Check sheet for the modelled part. Datum: model origin and axes. Units: mm. A direction names the side the tool comes from. Give positions to 0.01 mm unless a question says otherwise; leave off trailing zeros. Order: outer loops, then holes, each group sorted by start corner. A loop starts at its lowest first (then second) coordinate and runs counter-clockwise, first axis right, second up.
from build123d import *

# Parameters (mm, degrees)
SKETCH1_W            = 40
SKETCH1_H            = 20
BOSS_EXTRUDE1_DEPTH  = 35.9
SKETCH2_W            = 20
SKETCH2_H            = 2
BOSS_EXTRUDE2_DEPTH  = 7
SKETCH3_W            = 7
SKETCH3_H            = 1
BOSS_EXTRUDE3_DEPTH  = 1
CUT_EXTRUDE1_REACH   = 55.852
SKETCH4_R            = 2
FILLET1_R            = 1
CUT_EXTRUDE2_DEPTH   = 11
FILLET1_OF_MIRROR1_R = 1
SKETCH6_W            = 39
SKETCH6_H            = 19
BOSS_EXTRUDE4_DEPTH  = 0.5
BOSS_EXTRUDE5_DEPTH  = 2
SKETCH8_R            = 10
BOSS_EXTRUDE6_DEPTH  = 2.5
SKETCH9_R            = 6
BOSS_EXTRUDE7_DEPTH  = 1
SKETCH10_R           = 5
BOSS_EXTRUDE8_DEPTH  = 0.5
SKETCH11_W           = 10
SKETCH11_H           = 17
BOSS_EXTRUDE9_DEPTH  = 0.5
SKETCH12_R           = 3
BOSS_EXTRUDE10_DEPTH = 4
SKETCH13_W           = 6
SKETCH13_H           = 4
BOSS_EXTRUDE11_DEPTH = 1
SKETCH14_W           = 5.6
SKETCH14_H           = 3.6
SKETCH14_W_2         = 5
SKETCH14_H_2         = 3
BOSS_EXTRUDE12_DEPTH = 4


with BuildPart() as part:
    # Sketch1 → Boss-Extrude1 (new body)
    with BuildSketch(Plane(origin=(0, 0, 0), x_dir=(1, 0, 0), z_dir=(0, 1, 0))):
        with Locations((20, 10)):
            Rectangle(SKETCH1_W, SKETCH1_H)
    extrude(amount=BOSS_EXTRUDE1_DEPTH)

    # Sketch2 → Boss-Extrude2 (add)
    with BuildSketch(Plane(origin=(0, 0, 0), x_dir=(0, 0, -1), z_dir=(1, 0, 0))):
        with Locations((10, 29)):
            Rectangle(SKETCH2_W, SKETCH2_H)
    boss_extrude2 = extrude(amount=-BOSS_EXTRUDE2_DEPTH)

    # Sketch3 → Boss-Extrude3 (add)
    with BuildSketch(Plane(origin=(0, 30, 0), x_dir=(1, 0, 0), z_dir=(0, 1, 0))):
        with Locations((-3.5, 10)):
            Rectangle(SKETCH3_W, SKETCH3_H)
    boss_extrude3 = extrude(amount=BOSS_EXTRUDE3_DEPTH)

    # Sketch4 → Cut-Extrude1 (cut, up to next)
    with BuildSketch(Plane(origin=(0, 30, 0), x_dir=(1, 0, 0), z_dir=(0, 1, 0)), mode=Mode.PRIVATE) as cut_extrude1_sk1:
        with Locations((-5.2, 15.25)):
            Circle(SKETCH4_R)
    cut_extrude1_tool1 = extrude(cut_extrude1_sk1.sketch, amount=-CUT_EXTRUDE1_REACH, mode=Mode.PRIVATE) & part.part
    # Sketch4 → Cut-Extrude1 (cut, up to next)
    with BuildSketch(Plane(origin=(0, 30, 0), x_dir=(1, 0, 0), z_dir=(0, 1, 0)), mode=Mode.PRIVATE) as cut_extrude1_sk2:
        with Locations((-5.2, 4.75)):
            Circle(SKETCH4_R)
    cut_extrude1_tool2 = extrude(cut_extrude1_sk2.sketch, amount=-CUT_EXTRUDE1_REACH, mode=Mode.PRIVATE) & part.part
    cut_extrude1_1 = cut_extrude1_tool1.solids().sort_by_distance((-5.2, 30, -15.25))[0]
    add(cut_extrude1_1, mode=Mode.SUBTRACT)
    cut_extrude1_2 = cut_extrude1_tool2.solids().sort_by_distance((-5.2, 30, -4.75))[0]
    add(cut_extrude1_2, mode=Mode.SUBTRACT)
    cut_extrude1 = cut_extrude1_1 + cut_extrude1_2  # Cut-Extrude1 as one shape, for the pattern or mirror that repeats it

    # Fillet1
    fillet1_edges = [part.edges().sort_by_distance(p)[0] for p in [
        (-7, 29, 0),
        (-7, 29, -20),
    ]]
    fillet(fillet1_edges, radius=FILLET1_R)

    # Sketch5 → Cut-Extrude2 (cut)
    with BuildSketch(Plane.XY.offset(-9.5)):
        Polygon((-7, 30), (0, 31), (-7, 31), align=None)
    cut_extrude2 = extrude(amount=-CUT_EXTRUDE2_DEPTH, mode=Mode.SUBTRACT)

    # Mirror1: Boss-Extrude2, Boss-Extrude3, Cut-Extrude1, Cut-Extrude2 across plane
    add(boss_extrude2.mirror(Plane(origin=(20, 0, 0), x_dir=(0, 0, 1), z_dir=(1, 0, 0))))
    add(boss_extrude3.mirror(Plane(origin=(20, 0, 0), x_dir=(0, 0, 1), z_dir=(1, 0, 0))))
    add(cut_extrude1.mirror(Plane(origin=(20, 0, 0), x_dir=(0, 0, 1), z_dir=(1, 0, 0))), mode=Mode.SUBTRACT)
    add(cut_extrude2.mirror(Plane(origin=(20, 0, 0), x_dir=(0, 0, 1), z_dir=(1, 0, 0))), mode=Mode.SUBTRACT)

    # Fillet1 of Mirror1
    fillet1_of_mirror1_edges = [part.edges().sort_by_distance(p)[0] for p in [
        (47, 29, 0),
        (47, 29, -20),
    ]]
    fillet(fillet1_of_mirror1_edges, radius=FILLET1_OF_MIRROR1_R)

    # Sketch6 → Boss-Extrude4 (add)
    with BuildSketch(Plane(origin=(0, 35.9, 0), x_dir=(1, 0, 0), z_dir=(0, 1, 0))):
        with Locations((20, 10)):
            Rectangle(SKETCH6_W, SKETCH6_H)
    extrude(amount=BOSS_EXTRUDE4_DEPTH)

    # Sketch7 → Boss-Extrude5 (add)
    with BuildSketch(Plane(origin=(0, 36.4, 0), x_dir=(1, 0, 0), z_dir=(0, 1, 0))):
        with BuildLine():
            Line((5.5, 19.5), (30.5, 19.5))
            Line((30.5, 19.5), (30.5, 0.5))
            Line((30.5, 0.5), (5.5, 0.5))
            Line((5.5, 0.5), (5.5, 6.717431229))
            ThreePointArc((5.5, 6.717431229), (4.518757843, 10), (5.5, 13.282568771))
            Line((5.5, 13.282568771), (5.5, 19.5))
        make_face()
    extrude(amount=BOSS_EXTRUDE5_DEPTH)

    # Sketch8 → Boss-Extrude6 (add)
    with BuildSketch(Plane(origin=(0, 38.4, 0), x_dir=(1, 0, 0), z_dir=(0, 1, 0))):
        with Locations((30, 10)):
            Circle(SKETCH8_R)
    extrude(amount=-BOSS_EXTRUDE6_DEPTH)

    # Sketch9 → Boss-Extrude7 (add)
    with BuildSketch(Plane(origin=(0, 38.4, 0), x_dir=(1, 0, 0), z_dir=(0, 1, 0))):
        with Locations(Location((30, 10, 0), (0, 0, 270))):
            Circle(SKETCH9_R)
    extrude(amount=BOSS_EXTRUDE7_DEPTH)

    # Sketch10 → Boss-Extrude8 (add)
    with BuildSketch(Plane(origin=(0, 39.4, 0), x_dir=(1, 0, 0), z_dir=(0, 1, 0))):
        with Locations(Location((30, 10, 0), (0, 0, 270))):
            Circle(SKETCH10_R)
    extrude(amount=BOSS_EXTRUDE8_DEPTH)

    # Sketch11 → Boss-Extrude9 (add)
    with BuildSketch(Plane(origin=(0, 38.4, 0), x_dir=(1, 0, 0), z_dir=(0, 1, 0))):
        with BuildLine():
            Line((5.5, 0.5), (17.5, 0.5))
            Line((17.5, 0.5), (17.5, 8.5))
            ThreePointArc((17.5, 8.5), (19, 10), (17.5, 11.5))
            Line((17.5, 11.5), (17.5, 19.5))
            Line((17.5, 19.5), (5.5, 19.5))
            Line((5.5, 19.5), (5.5, 0.5))
        make_face()
        with Locations((11.5, 10)):
            Rectangle(SKETCH11_W, SKETCH11_H, mode=Mode.SUBTRACT)
    extrude(amount=BOSS_EXTRUDE9_DEPTH)

    # Sketch12 → Boss-Extrude10 (add)
    with BuildSketch(Plane(origin=(0, 39.9, 0), x_dir=(1, 0, 0), z_dir=(0, 1, 0))):
        with Locations(Location((30, 10, 0), (0, 0, 270))):
            Circle(SKETCH12_R)
    extrude(amount=BOSS_EXTRUDE10_DEPTH)

    # Sketch13 → Boss-Extrude11 (add)
    with BuildSketch(Plane(origin=(40, 0, 0), x_dir=(0, 0, -1), z_dir=(1, 0, 0))):
        with Locations((10, 5)):
            Rectangle(SKETCH13_W, SKETCH13_H)
    extrude(amount=BOSS_EXTRUDE11_DEPTH)

    # Sketch14 → Boss-Extrude12 (add)
    with BuildSketch(Plane(origin=(41, 0, 0), x_dir=(0, 0, -1), z_dir=(1, 0, 0))):
        with Locations((10, 5)):
            Rectangle(SKETCH14_W, SKETCH14_H)
        with Locations((10, 5)):
            Rectangle(SKETCH14_W_2, SKETCH14_H_2, mode=Mode.SUBTRACT)
    extrude(amount=BOSS_EXTRUDE12_DEPTH)


solid = part.part
1) Section check C-C, the plane x = 32. Record the cut outline in (y, z).
Recorded:
outline: (0, -20) - (35.9, -20) - (35.9, -19.8) - (38.4, -19.8) - (38.4, -15.66) - (39.4, -15.66) - (39.4, -14.58) - (39.9, -14.58) - (39.9, -12.24) - (43.9, -12.24) - (43.9, -7.76) - (39.9, -7.76) - (39.9, -5.42) - (39.4, -5.42) - (39.4, -4.34) - (38.4, -4.34) - (38.4, -0.2) - (35.9, -0.2) - (35.9, 0) - (0, 0) - close
2) Draft check along X on faces 1 (the face through (24.677, 38.893, -7.231)), 2 (the face through (37.9, 35.9, -0.2)), 3 (the face through (0, 33, -10)), 4 (the face through (19, 38.6, -10)). Enter one of: +X half, -X half, draft (parallel to the pull), parting line (faces both ways), or undercut.
Recorded:
face 1: undercut
face 2: draft
face 3: -X half
face 4: undercut
3) Set-up check for faces 5 (the face through (43, 5, -7.5)), 6 (the face through (43, 30, -5)), 7 (the face through (43, 5, -12.8)): record each of +Z, -Z, +X, -X, +Y, -Y from which the full face is reachable in a straight line by a thin tool's end or side.
Recorded:
face 5: +X
face 6: +Z, +X, +Y
face 7: -Z, +X, -Y
4) Section check A-A, the plane x = 38. Record the cut outline in (y, z).
Recorded:
outline: (0, -20) - (35.9, -20) - (35.9, -19.5) - (36.4, -19.5) - (36.4, -16) - (38.4, -16) - (38.4, -4) - (36.4, -4) - (36.4, -0.5) - (35.9, -0.5) - (35.9, 0) - (0, 0) - close
5) Material ranges on L1, parallel to Z at x = -5.2, y = 28.4; L2, parallel to Y at x = -0.5, z = -15.75; L3, parallel to Y at x = 17, z = -16.25, recorded low to high.
Recorded:
L1: z = -20 to -17.25, -13.25 to -6.75, -2.75 to 0
L2: y = 28 to 30
L3: y = 0 to 38.9
6) Section check D-D, the plane x = -2. Record the cut outline in (y, z).
Recorded:
outline: (28, -20) - (30, -20) - (30, -10.5) - (30.71, -10.5) - (30.71, -9.5) - (30, -9.5) - (30, 0) - (28, 0) - close
7) Section check B-B, the plane y = 14.5. Record the cut outline in (x, z), then the cut area to 3 significant figures.
Recorded:
outline: (0, -20) - (40, -20) - (40, 0) - (0, 0) - close
area: 800 mm2
8) Depth check by flat-ended pin: pin 1 Ø2 at (x, z) = (-2.5, -5) entering from +Y; pin 2 Ø7 at (x, z) = (35.5, -17) entering from +Y; pin 3 Ø2 at (y, z) = (17.5, -3) entering from -X. Enter the tip coordinate at first touch or a pass-through.
Recorded:
pin 1: stops at y = 30
pin 2: stops at y = 39.4
pin 3: stops at x = 0
